Work out the finished part from the listing and answer in its coordinate system (mm). A direction names the side the tool comes from. Coordinates: 2 decimals unless noted, no trailing zeros. Loops run counter-clockwise (first coordinate to the right, second up) from the corner with the lowest first, then second, coordinate; pieces in that order, holes last. Notation, with made-up numbers: (28, 63) -> (73, 63) arc R31 cw to (73, 88) -> close; hole circle Ø8 at (78, -15). An arc over 180 degrees is marked (long way). One line per question, with ' | ' between items.
```python
from build123d import *

# Parameters (mm, degrees)
SKETCH1_W               = 38.1
SKETCH1_H               = 38.1
SKETCH1_W_2             = 25.4
SKETCH1_H_2             = 25.4
EXTRUDE1_DEPTH          = 228.6
F_1_4_CLEARANCE_HOLE1_D = 6.7564
SKETCH4_W               = 12.7
SKETCH4_H               = 76.2
SKETCH4_W_2             = 38.1
SKETCH4_H_2             = 101.6
EXTRUDE2_DEPTH          = 3.175
SKETCH5_W               = 228.6
SKETCH5_H               = 38.1
EXTRUDE3_DEPTH          = 3.175
FILLET2_R               = 6.35
SKETCH8_W               = 76.2
SKETCH8_H               = 19.05
EXTRUDE6_DEPTH          = 232.579198116
FILLET3_R               = 6.35
FILLET4_R               = 6.35


with BuildPart() as part:
    # Sketch1 → Extrude1 (new body)
    with BuildSketch(Plane.XY):
        Rectangle(SKETCH1_W, SKETCH1_H)
        Rectangle(SKETCH1_W_2, SKETCH1_H_2, mode=Mode.SUBTRACT)
    extrude(amount=-EXTRUDE1_DEPTH)

    # 1/4 Clearance Hole1 (through all)
    with Locations(Plane(origin=(0, 19.05, 0), x_dir=(-1, 0, 0), z_dir=(0, 1, 0))):
        with Locations((0, -215.9), (0, -50.8), (0, -127)):
            Hole(F_1_4_CLEARANCE_HOLE1_D / 2)

    # Sketch4 → Extrude2 (cut)
    with BuildSketch(Plane(origin=(0, 19.05, 0), x_dir=(1, 0, 0), z_dir=(0, 1, 0))):
        with Locations((-12.7, 190.5)):
            Rectangle(SKETCH4_W, SKETCH4_H)
        with Locations((0, 50.8)):
            Rectangle(SKETCH4_W_2, SKETCH4_H_2)
        with Locations((12.7, 190.5)):
            Rectangle(SKETCH4_W, SKETCH4_H)
    extrude2 = extrude(amount=-EXTRUDE2_DEPTH, mode=Mode.SUBTRACT)

    # Mirror1: Extrude2 across plane
    add(extrude2.mirror(Plane.ZX), mode=Mode.SUBTRACT)

    # Sketch5 → Extrude3 (cut)
    with BuildSketch(Plane(origin=(19.05, 0, 0), x_dir=(0, 0, -1), z_dir=(1, 0, 0))):
        with Locations((114.3, 0)):
            Rectangle(SKETCH5_W, SKETCH5_H)
    extrude3 = extrude(amount=-EXTRUDE3_DEPTH, mode=Mode.SUBTRACT)

    # Mirror2: Extrude3 across plane
    add(extrude3.mirror(Plane(origin=(0, 0, 0), x_dir=(0, 0, 1), z_dir=(1, 0, 0))), mode=Mode.SUBTRACT)

    # Fillet2
    fillet2_edges = [part.edges().sort_by_distance(p)[0] for p in [
        (-6.35, 17.4625, -152.4),
        (6.35, 17.4625, -152.4),
    ]]
    fillet(fillet2_edges, radius=FILLET2_R)

    # Sketch8 → Extrude6 (cut, through all)
    with BuildSketch(Plane(origin=(15.875, 0, 0), x_dir=(0, 0, -1), z_dir=(1, 0, 0))):
        with Locations((190.5, -9.525)):
            Rectangle(SKETCH8_W, SKETCH8_H)
    extrude(amount=-EXTRUDE6_DEPTH, mode=Mode.SUBTRACT)

    # Fillet3
    fillet3_edges = [part.edges().sort_by_distance(p)[0] for p in [
        (-14.2875, 0, -152.4),
        (14.2875, 0, -152.4),
    ]]
    fillet(fillet3_edges, radius=FILLET3_R)

    # Fillet4
    fillet4_edges = [part.edges().sort_by_distance(p)[0] for p in [
        (-14.2875, 0, -228.6),
        (14.2875, 0, -228.6),
    ]]
    fillet(fillet4_edges, radius=FILLET4_R)


solid = part.part
```
1) For faces 4 (the face through (8.26, 17.44, -154.21)), 5 (the face through (-8.26, 17.44, -154.21)), 6 (the face through (-12.7, 0, -87)), 7 (the face through (-4, 15.875, -52)), determine the directions among +Z, -Z, +X, -X, +Y, -Y from which every point of the face is accessible in a straight line to the end or side of a thin tool.
Check values:
face 4: -Z, +X, +Y | face 5: -Z, -X, +Y | face 6: +Z, -Z | face 7: +Z, +X, -X, +Y
2) Find the intervals of material crossed by line 1 along Z through (x, y) = (0, 13); line 2 along Z through (x, y) = (0, 16.25); line 3 along Z through (x, y) = (0, -14.5), in increasing order.
Check values:
line 1: z = -228.6 to -219.28, -212.52 to -130.38, -123.62 to -54.18, -47.42 to 0 | line 2: z = -228.6 to -219.28, -212.52 to -130.38, -123.62 to -101.6 | line 3: z = -152.4 to -130.38, -123.62 to -54.18, -47.42 to 0
3) Find section A-A (x = 0). State how many separate pieces and enclosed holes the cut face has, plus the area to 3 significant figures.
Check values:
separate pieces: 7 | enclosed holes: 0 | area: 1,600 mm^2
4) Flat-ended cylindrical pins translate along their axes: pin 1 (7.5 mm diameter, centred on x = 12, z = -176.5, fed in from +Y) (3 decimals); pin 2 (2.5 mm diameter, centred on x = -15, z = -196, fed in from -Y); pin 3 (1.6 mm diameter, centred on x = 13.5, y = 18, fed in from -Z). Find the tip coordinate at first contact, or state that the pin passes through.
Check values:
pin 1: stops at y = 15.875 | pin 2: stops at y = 0 | pin 3: stops at z = -152.4
5) The mould has two halves that part along X. Classify faces 1 (the face through (-0.73, 14.27, -54.1)), 2 (the face through (-4, -15.875, -52)), 3 (the face through (15.875, 0, -113)): released by +X, released by -X, zero draft, split by the parting line, or undercut.
Check values:
face 1: undercut | face 2: zero draft | face 3: released by +X
6) Find section C-C (z = -78). Write down the section's boundary in (x, y) (3 decimals), plus the area to 3 significant figures.
Check values:
outline: (-15.875, -15.875) -> (15.875, -15.875) -> (15.875, 15.875) -> (-15.875, 15.875) -> close; hole (-12.7, -12.7) -> (12.7, -12.7) -> (12.7, 12.7) -> (-12.7, 12.7) -> close | area: 363 mm^2
7) Find section B-B (z = -50.8). Write down the section's boundary in (x, y) (3 decimals), plus the area to 3 significant figures.
Check values:
outline: (-15.875, -15.875) -> (-3.378, -15.875) -> (-3.378, -12.7) -> (-12.7, -12.7) -> (-12.7, 12.7) -> (-3.378, 12.7) -> (-3.378, 15.875) -> (-15.875, 15.875) -> close; (3.378, -15.875) -> (15.875, -15.875) -> (15.875, 15.875) -> (3.378, 15.875) -> (3.378, 12.7) -> (12.7, 12.7) -> (12.7, -12.7) -> (3.378, -12.7) -> close | area: 320 mm^2
8) Find section D-D (y = 4). Write down the section's boundary in (x, z) (3 decimals).
Check values:
outline: (-15.875, -228.149) -> (-12.7, -228.149) -> (-12.7, 0) -> (-15.875, 0) -> close; (12.7, -228.149) -> (15.875, -228.149) -> (15.875, 0) -> (12.7, 0) -> close
